Design review of the part built by this model. Coordinates are the model's own, in mm. A direction names the side the tool comes from. Coordinates: 2 decimals unless noted, no trailing zeros. Write each loop counter-clockwise with the first axis right and the second up, starting at its lowest first coordinate (ties: lowest second). Pieces come first, ordered by that corner, then holes.
Q1. Add section C-C, the plane x = -21. Give the boundary of the cut face in (y, z), plus the area to 3 significant figures.
Q2. Clearance check with flat-ended pins moving along their axes: pin 1 Ø0.6 at (y, z) = (1, -12) entering from -X; pin 2 Ø1 at (y, z) = (1.5, -14) entering from +X. State where each tip first meets the part, or that it passes through.
Q3. Machinability: for faces 1 (the face through (-43, 1, -7.75)), 2 (the face through (2.5, 1, 0)), 3 (the face through (42, 1, -7.75)), which of the approach directions +Z, -Z, +X, -X, +Y, -Y give a long, thin tool a straight path to every point of the face, cutting with its end or side? Answer none if there is none.
Q4. Add section A-A, the plane z = -13.25. Give the boundary of the cut face in (x, y).
Q5. Add section D-D, the plane x = 47.5. Give the boundary of the cut face in (y, z), plus the area to 3 significant figures.
Q6. To check wall thickness, follow probe 1 along X at (y, z) = (1.6, -6.25); probe 2 along X at (y, z) = (1.1, -3.75); probe 3 along Z at (x, y) = (5.5, 0.35). State the ranges of each line that lie inside material, in increasing order.
Q7. The part is to be moulded in two halves that separate along X. For faces 4 (the face through (-48.83, 0.99, 4.44)), 5 (the face through (55, 1, 0)), 6 (the face through (0, 1, -20.75)), say which applies: +X half, -X half, draft (parallel to the pull), parting line (faces both ways), or undercut.
Q8. Add section B-B, the plane x = 12. Give the boundary of the cut face in (y, z).
from build123d import *

# Parameters (mm, degrees)
SKETCH_1_R          = 1.5
SKETCH_1_R_2        = 1
EXTRUDE_1_DEPTH     = 2
SKETCH_2_W          = 16.25
SKETCH_2_H          = 6
SKETCH_2_W_2        = 23.5
SKETCH_2_H_2        = 7.5
CUT_EXTRUDE_1_DEPTH = 59.8180457
FILLET_1_R          = 1


with BuildPart() as part:
    # 草图1 → 凸台-拉伸1 (new body)
    with BuildSketch(Plane(origin=(0, 0, 0), x_dir=(1, 0, 0), z_dir=(0, 1, 0))):
        Polygon((30, 7.75), (55, 7.75), (55, -7.75), (-55, -7.75), (-55, 7.75), (-30, 7.75), (-30, 20.75), (30, 20.75), align=None)
        with Locations(Location((-47.5, 3.75, 0), (0, 0, 270))):
            Circle(SKETCH_1_R, mode=Mode.SUBTRACT)
        with Locations(Location((-47.5, -3.75, 0), (0, 0, 270))):
            Circle(SKETCH_1_R, mode=Mode.SUBTRACT)
        with Locations(Location((47.5, 3.75, 0), (0, 0, 270))):
            Circle(SKETCH_1_R, mode=Mode.SUBTRACT)
        with Locations(Location((47.5, -3.75, 0), (0, 0, 270))):
            Circle(SKETCH_1_R, mode=Mode.SUBTRACT)
        with Locations(Location((-12, 6.25, 0), (0, 0, 270))):
            Circle(SKETCH_1_R_2, mode=Mode.SUBTRACT)
        with Locations(Location((12, 6.25, 0), (0, 0, 270))):
            Circle(SKETCH_1_R_2, mode=Mode.SUBTRACT)
    extrude(amount=EXTRUDE_1_DEPTH)

    # 草图2 → 切除-拉伸1 (cut, through all)
    with BuildSketch(Plane(origin=(0, 2, 0), x_dir=(1, 0, 0), z_dir=(0, 1, 0))):
        with Locations((-31.875, 0.25)):
            Rectangle(SKETCH_2_W, SKETCH_2_H)
        with Locations((-10.625, 0.25)):
            Rectangle(SKETCH_2_W, SKETCH_2_H)
        with Locations((10.625, 0.25)):
            Rectangle(SKETCH_2_W, SKETCH_2_H)
        with Locations((31.875, 0.25)):
            Rectangle(SKETCH_2_W, SKETCH_2_H)
        with Locations((-14.25, 13)):
            Rectangle(SKETCH_2_W_2, SKETCH_2_H_2)
        with Locations((14.25, 13)):
            Rectangle(SKETCH_2_W_2, SKETCH_2_H_2)
    extrude(amount=-CUT_EXTRUDE_1_DEPTH, mode=Mode.SUBTRACT)

    # 圆角1
    fillet_1_edges = [part.edges().sort_by_distance(p)[0] for p in [
        (-40, 1, 2.75),
        (-40, 1, -3.25),
        (-23.75, 1, -3.25),
        (-23.75, 1, 2.75),
        (-55, 1, -7.75),
        (-30, 1, -7.75),
        (-30, 1, -20.75),
        (30, 1, -20.75),
        (30, 1, -7.75),
        (55, 1, -7.75),
        (55, 1, 7.75),
        (-55, 1, 7.75),
        (40, 1, 2.75),
        (23.75, 1, 2.75),
        (23.75, 1, -3.25),
        (40, 1, -3.25),
        (-26, 1, -9.25),
        (-26, 1, -16.75),
        (-2.5, 1, -16.75),
        (-2.5, 1, -9.25),
        (2.5, 1, -16.75),
        (26, 1, -16.75),
        (26, 1, -9.25),
        (2.5, 1, -9.25),
        (-18.75, 1, 2.75),
        (-18.75, 1, -3.25),
        (-2.5, 1, -3.25),
        (-2.5, 1, 2.75),
        (18.75, 1, -3.25),
        (18.75, 1, 2.75),
        (2.5, 1, 2.75),
        (2.5, 1, -3.25),
    ]]
    fillet(fillet_1_edges, radius=FILLET_1_R)


solid = part.part
Here are the results:
1. outline: (0, -20.75) - (2, -20.75) - (2, -16.75) - (0, -16.75) - close; (0, -9.25) - (2, -9.25) - (2, 7.75) - (0, 7.75) - close
1. area: 42.0 mm2
2. pin 1: stops at x = -30
2. pin 2: stops at x = 30
3. face 1: -Z, -X, +Y, -Y
3. face 2: +Y, -Y
3. face 3: -Z, +X, +Y, -Y
4. outline: (-30, 0) - (-26, 0) - (-26, 2) - (-30, 2) - close; (-2.5, 0) - (2.5, 0) - (2.5, 2) - (-2.5, 2) - close; (26, 0) - (30, 0) - (30, 2) - (26, 2) - close
5. outline: (0, -7.75) - (2, -7.75) - (2, -5.25) - (0, -5.25) - close; (0, -2.25) - (2, -2.25) - (2, 2.25) - (0, 2.25) - close; (0, 5.25) - (2, 5.25) - (2, 7.75) - (0, 7.75) - close
5. area: 19.0 mm2
6. probe 1: x = -55 to -13, -11 to 11, 13 to 55
6. probe 2: x = -55 to -49, -46 to 46, 49 to 55
6. probe 3: z = -20.75 to -16.75, -9.25 to -3.25, 2.75 to 7.75
7. face 4: undercut
7. face 5: +X half
7. face 6: draft
8. outline: (0, -20.75) - (2, -20.75) - (2, -16.75) - (0, -16.75) - close; (0, -9.25) - (2, -9.25) - (2, -7.25) - (0, -7.25) - close; (0, -5.25) - (2, -5.25) - (2, -3.25) - (0, -3.25) - close; (0, 2.75) - (2, 2.75) - (2, 7.75) - (0, 7.75) - close
